```python
from build123d import *

# Parameters (mm, degrees)
SKETCH1_W                = 42.3
SKETCH1_H                = 42.3
BOSS_EXTRUDE1_DEPTH      = 1
SKETCH2_W                = 42.3
SKETCH2_H                = 1
BOSS_EXTRUDE2_DEPTH      = 10
CUT_EXTRUDE2_DEPTH       = 1
CUT_EXTRUDE4_DEPTH       = 10
MIRROR2_COPY_1_DEPTH     = 1
CHAMFER1_SIZE            = 5
SKETCH8_W                = 42.3
SKETCH8_H                = 1
BOSS_EXTRUDE3_DEPTH      = 27
BOSS_EXTRUDE3_DEPTH_BACK = 1
SKETCH5_R                = 3
CUT_EXTRUDE3_DEPTH       = 22
CUT_EXTRUDE5_REACH       = 44.3
SKETCH9_W                = 10
SKETCH9_H                = 1
BOSS_EXTRUDE4_DEPTH      = 9
SKETCH11_R               = 2
CUT_EXTRUDE6_DEPTH       = 10
SKETCH15_R               = 3
CUT_EXTRUDE8_DEPTH       = 10


with BuildPart() as part:
    # Sketch1 → Boss-Extrude1 (new body)
    with BuildSketch(Plane.XY):
        Rectangle(SKETCH1_W, SKETCH1_H)
    extrude(amount=BOSS_EXTRUDE1_DEPTH)

    # Sketch2 → Boss-Extrude2 (add)
    with BuildSketch(Plane.XY.offset(1)):
        with Locations((0, -20.65)):
            Rectangle(SKETCH2_W, SKETCH2_H)
    extrude(amount=BOSS_EXTRUDE2_DEPTH)

    # Sketch3 → Cut-Extrude2 (cut)
    with BuildSketch(Plane.XY.offset(1)):
        with BuildLine():
            Line((-15.470931569, -14.025299874), (-12.470931569, -14.025299874))
            ThreePointArc((-12.470931569, -14.025299874), (-10.970931569, -15.525299874), (-12.470931569, -17.025299874))
            Line((-12.470931569, -17.025299874), (-15.470931569, -17.025299874))
            ThreePointArc((-15.470931569, -17.025299874), (-16.970931569, -15.525299874), (-15.470931569, -14.025299874))
        make_face()
    cut_extrude2 = extrude(amount=-CUT_EXTRUDE2_DEPTH, mode=Mode.SUBTRACT)

    # Mirror1: Cut-Extrude2 across plane
    add(cut_extrude2.mirror(Plane(origin=(0, 0, 0), x_dir=(0, 0, 1), z_dir=(1, 0, 0))), mode=Mode.SUBTRACT)

    # Sketch6 → Cut-Extrude4 (cut)
    with BuildSketch(Plane.XY.offset(1)):
        with BuildLine():
            Line((10, 3.5), (10, -3.5))
            ThreePointArc((10, -3.5), (0, -13.5), (-10, -3.5))
            Line((-10, -3.5), (-10, 3.5))
            ThreePointArc((-10, 3.5), (0, 13.5), (10, 3.5))
        make_face()
    extrude(amount=-CUT_EXTRUDE4_DEPTH, mode=Mode.SUBTRACT)

    # Mirror2: Cut-Extrude2 across plane
    add(cut_extrude2.mirror(Plane.ZX), mode=Mode.SUBTRACT)

    # Mirror2 copy 1 sketch → Mirror2 copy 1 (cut)
    with BuildSketch(Plane(origin=(0, 0, 1), x_dir=(-1, 0, 0), z_dir=(0, 0, 1))):
        with BuildLine():
            Line((-15.470931569, -14.025299874), (-12.470931569, -14.025299874))
            ThreePointArc((-12.470931569, -14.025299874), (-10.970931569, -15.525299874), (-12.470931569, -17.025299874))
            Line((-12.470931569, -17.025299874), (-15.470931569, -17.025299874))
            ThreePointArc((-15.470931569, -17.025299874), (-16.970931569, -15.525299874), (-15.470931569, -14.025299874))
        make_face()
    extrude(amount=-MIRROR2_COPY_1_DEPTH, mode=Mode.SUBTRACT)

    # Chamfer1
    chamfer1_edges = [part.edges().sort_by_distance(p)[0] for p in [
        (-21.15, 21.15, 0.5),
        (21.15, 21.15, 0.5),
    ]]
    chamfer(chamfer1_edges, length=CHAMFER1_SIZE)

    # Sketch8 → Boss-Extrude3 (add, two sides)
    with BuildSketch(Plane(origin=(0, 0, 0), x_dir=(-1, 0, 0), z_dir=(0, 0, -1))) as boss_extrude3_sk:
        with Locations((0, -21.65)):
            Rectangle(SKETCH8_W, SKETCH8_H)
    extrude(amount=BOSS_EXTRUDE3_DEPTH)
    extrude(boss_extrude3_sk.sketch, amount=-BOSS_EXTRUDE3_DEPTH_BACK)

    # Sketch5 → Cut-Extrude3 (cut)
    with BuildSketch(Plane(origin=(0, -20.15, 0), x_dir=(1, 0, 0), z_dir=(0, 1, 0))):
        with Locations((0, -6)):
            Circle(SKETCH5_R)
    extrude(amount=-CUT_EXTRUDE3_DEPTH, mode=Mode.SUBTRACT)

    # Sketch9 → Cut-Extrude5 (cut, up to next)
    with BuildSketch(Plane(origin=(21.15, 0, 0), x_dir=(0, 0, -1), z_dir=(1, 0, 0)), mode=Mode.PRIVATE) as cut_extrude5_sk1:
        with Locations((-6, -20.65)):
            Rectangle(SKETCH9_W, SKETCH9_H)
    cut_extrude5_tool1 = extrude(cut_extrude5_sk1.sketch, amount=-CUT_EXTRUDE5_REACH, mode=Mode.PRIVATE) & part.part
    add(cut_extrude5_tool1.solids().sort_by_distance((21.15, -20.65, 6))[0], mode=Mode.SUBTRACT)

    # Sketch10 → Boss-Extrude4 (add)
    with BuildSketch(Plane(origin=(21.15, 0, 0), x_dir=(0, 0, -1), z_dir=(1, 0, 0))):
        Polygon((0, -21.15), (-1, -21.15), (-1, -22.15), (0, -22.15), (27, -22.15), (27, -21.15), align=None)
    boss_extrude4 = extrude(amount=BOSS_EXTRUDE4_DEPTH)

    # Mirror3: Boss-Extrude4 across plane
    add(boss_extrude4.mirror(Plane(origin=(0, 0, 0), x_dir=(0, 0, 1), z_dir=(1, 0, 0))))

    # Sketch11 → Cut-Extrude6 (cut)
    with BuildSketch(Plane(origin=(0, -21.15, 0), x_dir=(1, 0, 0), z_dir=(0, 1, 0))):
        with Locations((26, 13)):
            Circle(SKETCH11_R)
        with Locations((-26, 13)):
            Circle(SKETCH11_R)
    extrude(amount=-CUT_EXTRUDE6_DEPTH, mode=Mode.SUBTRACT)

    # Sketch15 → Cut-Extrude8 (cut)
    with BuildSketch(Plane(origin=(0, -21.15, 0), x_dir=(1, 0, 0), z_dir=(0, 1, 0))):
        with Locations((0, 20)):
            Circle(SKETCH15_R)
    extrude(amount=-CUT_EXTRUDE8_DEPTH, mode=Mode.SUBTRACT)


solid = part.part
```
The listing builds one solid part. Answer for the finished solid, in the listing's coordinates (mm). A direction names the side the tool comes from. Coordinates: 2 decimals unless noted, no trailing zeros. Order: outer loops, then holes, each group sorted by start corner. A loop starts at its lowest first (then second) coordinate and runs counter-clockwise, first axis right, second up. Notation, with made-up numbers: M 5.25,3 L 45.25,3 A14 ccw 45.25,30 Z; hole C 30.25,8 d11. An arc over 180 degrees is marked long. Answer as a JSON object with one key per item and string values. Group by question number.
1. Flat-ended cylindrical pins translate along their axes: P1, Ø5, axis at x = 26, z = -13, coming from the -Y side; P2, Ø10, axis at y = -15, z = -22, coming from the +X side; P3, Ø8, axis at x = -11, y = -2, coming from the -Z side; P4, Ø4.5, axis at x = -26, z = -13, coming from the +Y side. Find the tip coordinate at first contact, or state that the pin passes through.
2. Section D-D on x = 0 is taken. Write down the section's boundary in (y, z), then the cut area to 3 significant figures.
3. A tool of negligible diameter and unlimited length cuts with its end or side. For faces 5 (the cylindrical face through (16.97, -15.56, 0.51)), 6 (the flat face through (-10, -9, 0)), 7 (the flat face through (14, 0, 1)), from which of +Z, -Z, +X, -X, +Y, -Y can it reach the whole face along a straight path? Write none if from no direction.
4. Straight lines are drawn through the part: line 1 (Z direction, x = 0, y = -21.85); line 2 (X direction, y = -21.55, z = -13); line 3 (Z direction, x = -26, y = -21.4). For each, find the intervals that lie inside material, in ascending order.
5. Determine the mould class of faces 1 (the cylindrical face through (-26.26, -21.643, -14.983)), 2 (the flat face through (0, -22.15, -13)), 3 (the cylindrical face through (10.97, -15.49, 0.51)), 4 (the flat face through (18.7, 18.6, 0.5)) for opening direction Y: released by +Y, released by -Y, zero draft, split by the parting line, or undercut.
6. Section B-B on z = -20 is taken. Write down the section's boundary in (x, y).
7. Section C-C on y = -0.5 is taken. Write down the section's boundary in (x, z), then the cut area to 3 significant figures.
8. Section A-A on x = -8 is taken. Write down the section's boundary in (y, z), then the cut area to 3 significant figures.
Values follow:
{
 "1": {"P1": "y = -22.15", "P2": "through", "P3": "z = 0", "P4": "y = -21.15"},
 "2": {"outline": "M -22.15,-27 L -21.15,-27 L -21.15,-23 L -22.15,-23 Z; M -22.15,-17 L -21.15,-17 L -21.15,0 L -13.5,0 L -13.5,1 L -22.15,1 Z; M 13.5,0 L 21.15,0 L 21.15,1 L 13.5,1 Z", "area": "37.3 mm2"},
 "3": {"face 5": "+Z, -Z", "face 6": "-Z, +X, -X, +Y", "face 7": "+Z, +X, -X, +Y, -Y"},
 "4": {"line 1": "-27 to -23, -17 to 1", "line 2": "-30.15 to -28, -24 to 24, 28 to 30.15", "line 3": "-27 to -15, -11 to 1"},
 "5": {"face 1": "zero draft", "face 2": "released by -Y", "face 3": "undercut", "face 4": "released by +Y"},
 "6": {"outline": "M -30.15,-22.15 L -3,-22.15 L -3,-21.15 L -30.15,-21.15 Z; M 3,-22.15 L 30.15,-22.15 L 30.15,-21.15 L 3,-21.15 Z"},
 "7": {"outline": "M -21.15,0 L -10,0 L -10,1 L -21.15,1 Z; M 10,0 L 21.15,0 L 21.15,1 L 10,1 Z", "area": "22.3 mm2"},
 "8": {"outline": "M -22.15,-27 L -21.15,-27 L -21.15,0 L -9.5,0 L -9.5,1 L -22.15,1 Z; M 9.5,0 L 21.15,0 L 21.15,1 L 9.5,1 Z", "area": "51.3 mm2"}
}
